Could you check a few things on this model? Use its own coordinates, in mm. Face numbers are marked on the shaded views. A direction names the side the tool comes from. Give positions to 0.01 mm unless a question says otherwise; leave off trailing zeros. Order: outer loops, then holes, each group sorted by start corner. A loop starts at its lowest first (then second) coordinate and runs counter-clockwise, first axis right, second up. Notation, with made-up numbers: M 26,-31 L 43,-31 A18 cw 43,-25 Z; hole C -24,-32 d2. An arc over 180 degrees is marked long. Use a Markdown table: item, result. Add a question column.
Item 1: If I drill on L1, parallel to X at y = -1078.5, z = -13.75; L2, parallel to Z at x = 811, y = -678; L3, parallel to X at y = -1253.5, z = -1.5, over which ranges is the centre line in solid material (lowest first)? Write a range as from..to.
Item 2: I'm going to push flat-ended pins straight in: pin 1 Ø1.6 at (y, z) = (-879, 1.5) entering from +X; pin 2 Ø4.5 at (y, z) = (-675.5, -10) entering from -X; pin 3 Ø1 at (x, y) = (842.5, -845.5) entering from -Z. Where does each tip first touch, or does it pass through?
Item 3: Suppose I cut it at C-C on y = -1213. Write out the boundary of the cut face in (x, z).
Item 4: Suppose I cut it at D-D on y = -548. Write out the boundary of the cut face in (x, z), plus the area to 3 significant figures.
Item 5: For the marked faces 1 and 2, which set-ups out of +Z, -Z, +X, -X, +Y, -Y let a thin tool reach every point of the face, with its end or its side?
Item 6: Suppose I cut it at A-A on z = -6.5. Write out the boundary of the cut face in (x, y), plus the area to 3 significant figures.
Item 7: Suppose I cut it at B-B on x = 830.5. Write out the boundary of the cut face in (y, z), plus the area to 3 significant figures.
Autodesk Inventor part; units mm, degrees
ref_plane "YZ Plane" through (0, 0, 0) normal (1, 0, 0) x (0, 1, 0)
ref_plane "XZ Plane" through (0, 0, 0) normal (0, 1, 0) x (-1, 0, 0)
ref_plane "XY Plane" through (0, 0, 0) normal (0, 0, 1) x (1, 0, 0)
sketch "Sketch1" plane through (0, 0, 0) normal (0, 0, 1) x (1, 0, 0)
  arc A0 (750, -2100) -> (770.3488, -241.0426) centre (-10250, -1050) ccw construction
  arc A1 (752.9864, -2100.2851) -> (771.4818, -215.8854) centre (-10246.9892, -1050.0296) ccw
  line L0 (-750, -2700) -> (-750, 0) construction
  line L1 (-800, 50) -> (-800, -2750) construction
  line L2 (-850, -2800) -> (-850, 100) construction
  line L3 (850, 100) -> (850, -2800)
  line L4 (800, -2750) -> (800, 50) construction
  line L5 (750, 0) -> (750, -2700) construction
  line L6 (770.3488, -241.0426) -> (767.3569, -241.2622) construction
  line L7 (768.4904, -216.1118) -> (771.4818, -215.8854) construction
  arc A2 (747.4657, -5.0326) -> (744.8748, -2.3426) centre (744.4792, -5.3164) ccw construction
  arc A3 (747.4657, -5.0326) -> (747.0136, -0.2851) centre (-10252.9895, -1050.2524) ccw construction
  arc A4 (767.3569, -241.2622) -> (747.4657, -5.0326) centre (-10252.9895, -1050.2524) ccw construction
  line L8 (750, 0) -> (747.0136, -0.2851) construction
  arc A5 (750.4522, -4.7486) -> (750, 0) centre (-10250, -1050) ccw construction
  arc A6 (750.4522, -4.7486) -> (745.2706, 0.6314) centre (744.4791, -5.3162) ccw
  line L9 (-750, 0) -> (750, 0) construction
  line L10 (-850, 100) -> (850, 100) construction
  line L11 (800, 50) -> (-800, 50) construction
  arc A7 (770.3488, -241.0426) -> (750.4522, -4.7486) centre (-10250, -1050) ccw
  line L12 (750, -2700) -> (-750, -2700) construction
  line L13 (750, -2100) -> (752.9864, -2100.2851) construction
  line L14 (-800, -2750) -> (800, -2750)
  line L15 (850, -2800) -> (-850, -2800) construction
  arc A8 (110, -2700) -> (114.1118, -2698.3696) centre (110, -2694) ccw construction
  line L16 (0, -2697) -> (110, -2697) construction
  line L17 (0, -2700) -> (0, -2697) construction
  arc A9 (750, 0) -> (745.2706, 0.6314) centre (0, -5600) ccw construction
  line L18 (750, 0) -> (749.6018, -2.9735) construction
  arc A10 (750, -3.0268) -> (0, 47) centre (-0.2, -5603) ccw construction
  line L19 (0, 47) -> (0, 0) construction
  line L20 (0, 50) -> (0, 47) construction
  line L21 (0, 100) -> (0, 50)
  arc A11 (745.2706, 0.6314) -> (0, 50) centre (0, -5600) ccw construction
  line L22 (-750, -2100) -> (750, -2100) construction
  arc A12 (110, -2697) -> (112.0559, -2696.1848) centre (110, -2694) ccw construction
  line L23 (676.3163, -2173.4556) -> (674.2605, -2171.2708) construction
  line L24 (690.4112, -2151.9536) -> (692.4671, -2154.1384) construction
  line L25 (752.0559, -2102.1848) -> (676.3163, -2173.4556) construction
  line L26 (114.1118, -2698.3696) -> (750, -2100) construction
  arc A13 (752.0559, -2102.1848) -> (752.9864, -2100.2851) centre (749.9998, -2099.9999) ccw construction
  line L27 (750, -2100) -> (752.0559, -2102.1848) construction
  arc A14 (749.1768, -2100.7746) -> (750.1074, -2098.8746) centre (747.1209, -2098.5898) ccw construction
  line L28 (112.0559, -2696.1848) -> (690.4112, -2151.9536) construction
  line L29 (850, -261.0426) -> (774.8074, -261.0426)
  arc A15 (800, 50) -> (0, 100) centre (0, -6325) ccw construction
  arc A16 (824.8074, -261.0426) -> (800, 50) centre (-10695.3477, -1023.3288) ccw construction
  line L30 (824.8074, -261.0426) -> (824.8074, 100) construction
  arc A17 (789.9065, -2131.1044) -> (824.8074, -261.0426) centre (-10201.0809, -990.6233) ccw construction
  line L31 (0, -2700) -> (0, -2750) construction
  line L32 (112.3791, -2700) -> (132.2053, -2750) construction
  line L33 (132.2053, -2750) -> (850, -2074.5565)
  arc A18 (770.2924, -241.0467) -> (766.5756, -191.1852) centre (768.4904, -216.1118) ccw construction
  line L34 (850, -400) -> (783.8749, -400) construction
  line L35 (850, -900) -> (801.9923, -900) construction
  line L36 (850, -1400) -> (797.4674, -1400) construction
  line L37 (850, -1900) -> (770.2723, -1900) construction
  line L38 (350, 100) -> (350, 39.1489)
  line L39 (-1472.612, -150) -> (-973.4947, -150)
  line L40 (-1472.612, -700) -> (-973.4947, -700)
  line L41 (-1472.612, -1250) -> (-973.4947, -1250)
  line L42 (-1472.612, -1800) -> (-973.4947, -1800)
  line L43 (800, -2750) -> (850, -2750) construction
  line L44 (752.9864, -2100.2851) -> (850, -2100.2851)
  point P0 (822.6583, -2100.2851)
  dimension "d16" = 1500
  dimension "d17" = 2700
  dimension "d18" = 2100
  dimension "d19" = 6
  dimension "d20" = 3
  dimension "d21" = 3
  dimension "d22" = 6
  dimension "d23" = 3
  dimension "d24" = 241.9
  dimension "d25" = 50
  dimension "d26" = 50
  dimension "d27" = 3
  dimension "d28" = 110
  dimension "d29" = 25
  dimension "d30" = 104
  dimension "d31" = 25
  dimension "d32" = 20
  dimension "d33" = 50
  dimension "d57" = 500
  dimension "d58" = 500
  dimension "d59" = 500
  dimension "d60" = 500
  dimension "d61" = 500
  dimension "d83" = 250
  dimension "d86" = 550
  dimension "d91" = 274.5565
extrude "Plate3" add sketch "Sketch1" along normal blind 2
sketch "Sketch3" plane through (848, -261.0426, 2) normal (1, 0, 0) x (0, 1, 0)
  line L0 (-1839.2425, 0) -> (0, 0)
  line L1 (0, 0) -> (0, 20)
  line L2 (0, 20) -> (-1839.2425, 20)
  line L3 (-1839.2425, 20) -> (-1839.2425, 0)
edge flange "Flange2" height 20 angle 90 thickness 2 bend radius 2.75 thickness toward (1, 0, 0) relief round relief width 2 relief depth 1 edges at (850, -1167.7996, 2) wall of the first edge with corners at (848, -2100.2851, 2) (848, -261.0426, 2) (848, -261.0426, -18) (848, -2100.2851, -18)
bend "Bend2"
corner "Corner2"
sketch "Sketch5" plane through (0, 0, 0) normal (0, 0, 1) x (1, 0, 0)
  line L0 (845.25, -2100.2851) -> (845.25, -261.0426)
  line L1 (774.8074, -261.0426) -> (845.25, -261.0426)
  arc A0 (752.9864, -2100.2851) -> (774.8074, -261.0426) centre (-10246.9892, -1050.0296) ccw
  line L2 (850, -261.0426) -> (850, -2100.2851)
  line L3 (850, -376.0426) -> (819, -376.0426)
  line L4 (850, -378.0426) -> (848, -378.0426) construction
  line L5 (848, -2100.2851) -> (848, -261.0426)
  line L6 (819, -376.0426) -> (819, -378.0426)
  line L7 (850, -876.0416) -> (801.641, -876.0416) construction
  line L8 (850, -878.0416) -> (801.6723, -878.0416) construction
  line L9 (820, -876.0416) -> (820, -878.0416) construction
  line L10 (850, -1376.0416) -> (798.2005, -1376.0416) construction
  line L11 (850, -1378.0416) -> (798.1413, -1378.0416) construction
  line L12 (820, -1376.0416) -> (820, -1378.0416) construction
  line L13 (850, -1876.0416) -> (772.0945, -1876.0416) construction
  line L14 (850, -1878.0416) -> (771.9443, -1878.0416) construction
  line L15 (820, -1876.0416) -> (820, -1878.0416) construction
  line L16 (850, -881.0416) -> (845.25, -881.0416) construction
  line L17 (845.25, -1381.0416) -> (850, -1381.0416) construction
  line L18 (845.25, -1881.0416) -> (850, -1881.0416) construction
  line L19 (845.25, -2100.2851) -> (752.9864, -2100.2851)
  line L20 (850, -376.0426) -> (850, -381.0426)
  line L21 (848, -376.0426) -> (848, -378.0426) construction
  line L22 (850, -381.0426) -> (848, -381.0426)
  line L23 (819, -376.0426) -> (782.437, -376.0426) construction
  line L24 (819, -378.0426) -> (782.559, -378.0426) construction
  line L25 (848, -378.0426) -> (848, -381.0426)
  line L26 (848, -378.0426) -> (819, -378.0426)
  line L27 (848, -381.0426) -> (845.25, -381.0426)
  point P0 (0, 0)
  point P1 (845.25, -380.4205)
  point P2 (848, -380.4205)
  point P3 (848, -1881.0416)
  point P4 (848, -1878.0416)
  point P5 (848, -1381.0416)
  point P6 (848, -1378.0416)
  point P7 (848, -881.0416)
  point P8 (848, -878.0416)
  point P9 (819, -377.0426)
  point P10 (848, -381.0426)
  point P11 (850, -410.4205)
  point P12 (848, -376.0426)
  point P13 (820, -877.0416)
  point P14 (820, -1377.0416)
  point P15 (820, -1877.0416)
  point P16 (848, -381.0426)
  point P17 (845.25, -378.0426)
  dimension "d69" = 1839.2425
  dimension "d70" = 2
  dimension "d76" = 67.563
  dimension "d80" = 48.359
  dimension "d81" = 30
  dimension "d94" = 5
  dimension "d95" = 30
  dimension "d96" = 5
  dimension "d97" = 30
  dimension "d98" = 5
  dimension "d102" = 77.9056
  dimension "d104" = 51.7995
  dimension "d106" = 2
  dimension "d107" = 5
  dimension "d108" = 116
  dimension "d109" = 500
  dimension "d110" = 500
  dimension "d111" = 500
  dimension "d112" = 31
extrude "Extrusion2" cut sketch "Sketch5" along normal through all both and the other way through all contours L0 L26 L5 L27 | L26 L6 L3 L0 | L0 L3 L5 L26 | L5 L3 L2 L22
chamfer "Chamfer2" [suppressed]
pattern_linear "Rectangular Pattern3" count 4 spacing 500 along (0, -1, 0) of "Extrusion2"
sketch "Sketch6" plane through (0, 0, 0) normal (0, 0, -1) x (-1, 0, 0)
  line L0 (-803.1643, -1276.0426) -> (-817.1643, -1276.0426) construction
  line L1 (-817.1643, -1276.0426) -> (-817.1643, -1076.0426) construction
  line L2 (-817.1643, -1076.0426) -> (-803.1643, -1076.0426) construction
  line L3 (-803.1643, -1076.0426) -> (-803.1643, -1276.0426) construction
  line L4 (-752.9864, -2100.2851) -> (-845.25, -2100.2851)
  line L5 (-803.1643, -1801.0426) -> (-803.1643, -1851.0426) construction
  line L6 (-803.1643, -1851.0426) -> (-815.1643, -1851.0426) construction
  line L7 (-815.1643, -1851.0426) -> (-815.1643, -1801.0426) construction
  line L8 (-815.1643, -1801.0426) -> (-803.1643, -1801.0426) construction
  line L9 (-845.25, -1876.0426) -> (-819, -1876.0426)
  line L10 (-803.1643, -1301.0426) -> (-803.1643, -1351.0426) construction
  line L11 (-803.1643, -1351.0426) -> (-815.1643, -1351.0426) construction
  line L12 (-815.1643, -1351.0426) -> (-815.1643, -1301.0426) construction
  line L13 (-815.1643, -1301.0426) -> (-803.1643, -1301.0426) construction
  line L14 (-803.1643, -801.0426) -> (-803.1643, -851.0426) construction
  line L15 (-803.1643, -851.0426) -> (-815.1643, -851.0426) construction
  line L16 (-815.1643, -851.0426) -> (-815.1643, -801.0426) construction
  line L17 (-815.1643, -801.0426) -> (-803.1643, -801.0426) construction
  line L18 (-803.1643, -301.0426) -> (-803.1643, -351.0426) construction
  line L19 (-803.1643, -351.0426) -> (-815.1643, -351.0426) construction
  line L20 (-815.1643, -351.0426) -> (-815.1643, -301.0426) construction
  line L21 (-815.1643, -301.0426) -> (-803.1643, -301.0426) construction
  line L22 (-845.25, -1376.0426) -> (-819, -1376.0426)
  line L23 (-845.25, -876.0426) -> (-819, -876.0426)
  line L24 (-845.25, -376.0426) -> (-819, -376.0426)
  point P0 (0, 0)
  point P1 (-753.1643, -2098.4205)
  point P2 (-824.6397, -2098.4205)
  dimension "d120" = 200
  dimension "d121" = 14
  dimension "d124" = 50
  dimension "d125" = 12
  dimension "d126" = 50
  dimension "d127" = 25
  dimension "d128" = 50
  dimension "d129" = 12
  dimension "d130" = 50
  dimension "d131" = 12
  dimension "d132" = 50
  dimension "d133" = 12
  dimension "d134" = 50
  dimension "d135" = 25
  dimension "d136" = 25
  dimension "d137" = 25
  dimension "d138" = 50
  dimension "d139" = 50
  dimension "d140" = 50
  dimension "d143" = 100
mark "Mark1"
sketch "Sketch7" plane through (0, 0, 0) normal (0, 0, 1) x (1, 0, 0)
  line L0 (845.25, -1878.0426) -> (819, -1878.0426) construction
  line L1 (819, -1878.0426) -> (819, -1876.0426) construction
  line L2 (819, -1876.0426) -> (845.25, -1876.0426) construction
  line L3 (845.25, -1876.0426) -> (845.25, -1381.0426) construction
  line L4 (845.25, -1381.0426) -> (845.25, -1378.0426) construction
  line L5 (845.25, -1378.0426) -> (819, -1378.0426) construction
  line L6 (819, -1378.0426) -> (819, -1376.0426) construction
  line L7 (819, -1376.0426) -> (845.25, -1376.0426) construction
  line L8 (845.25, -1376.0426) -> (845.25, -881.0426) construction
  line L9 (845.25, -881.0426) -> (845.25, -878.0426) construction
  line L10 (845.25, -878.0426) -> (819, -878.0426) construction
  line L11 (819, -878.0426) -> (819, -876.0426) construction
  line L12 (819, -876.0426) -> (845.25, -876.0426) construction
  line L13 (845.25, -876.0426) -> (845.25, -381.0426) construction
  line L14 (845.25, -381.0426) -> (845.25, -378.0426)
  line L15 (845.25, -378.0426) -> (819, -378.0426)
  line L16 (819, -378.0426) -> (819, -376.0426)
  line L17 (819, -376.0426) -> (845.25, -376.0426)
  line L18 (845.25, -376.0426) -> (845.25, -261.0426)
  line L19 (774.8074, -261.0426) -> (845.25, -261.0426)
  arc A0 (752.9864, -2100.2851) -> (774.8074, -261.0426) centre (-10246.9892, -1050.0296) ccw construction
  line L20 (845.25, -2100.2851) -> (752.9864, -2100.2851) construction
  line L21 (845.25, -2100.2851) -> (845.25, -1881.0426) construction
  line L22 (845.25, -1881.0426) -> (845.25, -1878.0426) construction
  line L23 (716.6808, -2132.1957) -> (990.5996, -2132.1957)
  line L24 (990.5996, -2132.1957) -> (990.5996, -1376.0426)
  line L25 (990.5996, -1376.0426) -> (716.6808, -1376.0426)
  line L26 (716.6808, -1376.0426) -> (716.6808, -2132.1957)
  point P0 (0, 0)
extrude "Extrusion3" cut sketch "Sketch7" along normal through all both and the other way through all
equation "\"d16\" = d34"
equation "\"d17\" = d35"
equation "\"d18\" = d36"
equation "\"d19\" = d37"
equation "\"d20\" = d38"
equation "\"d21\" = d39"
equation "\"d22\" = d39 + d43"
equation "\"d23\" = d39"
equation "\"d27\" = d39"
equation "\"d28\" = 0.5 * d44"
equation "\"d29\" = d41"
equation "\"d30\" = d42"
equation "\"d31\" = d41"
equation "\"d33\" = d25"
equation "\"Стрингер_3\" = 67.36301"
equation "\"d37\" = d39 + d43"
equation "\"d38\" = d39"
equation "\"d43\" = d39"
equation "\"Стрингер_4\" = 48.15903"
equation "\"Стрингер_5\" = 51.59945"
equation "\"Стрингер_6\" = 77.70555"
properties part number "MSC 315 rib hip" material "Stainless Steel"
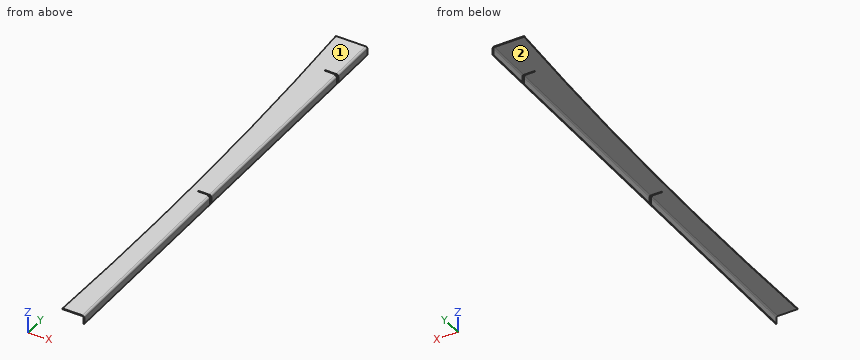
Findings below:
| question | item | result |
|---|---|---|
| 1 | L1 | x = 848..850 |
| 1 | L2 | z = 0..2 |
| 1 | L3 | x = 847.7..849.83 |
| 2 | pin 1 | stops at x = 845.25 |
| 2 | pin 2 | stops at x = 848 |
| 2 | pin 3 | stops at z = 0 |
| 3 | outline | M 801.81,0 L 845.25,0 A2.75 cw 848,-2.75 L 848,-18 L 850,-18 L 850,-2.75 A4.75 ccw 845.25,2 L 801.81,2 Z |
| 4 | outline | M 791.6,0 L 845.25,0 A2.75 cw 848,-2.75 L 848,-18 L 850,-18 L 850,-2.75 A4.75 ccw 845.25,2 L 791.6,2 Z |
| 4 | area | 150 mm^2 |
| 5 | face 1 | +Z, +X, -X, +Y, -Y |
| 5 | face 2 | -Z, -X, +Y, -Y |
| 6 | outline | M 848,-1376.04 L 850,-1376.04 L 850,-881.04 L 848,-881.04 Z; M 848,-876.04 L 850,-876.04 L 850,-381.04 L 848,-381.04 Z; M 848,-376.04 L 850,-376.04 L 850,-261.04 L 848,-261.04 Z |
| 6 | area | 2,210 mm^2 |
| 7 | outline | M -1376.04,0 L -878.04,0 L -878.04,2 L -1376.04,2 Z; M -876.04,0 L -378.04,0 L -378.04,2 L -876.04,2 Z; M -376.04,0 L -261.04,0 L -261.04,2 L -376.04,2 Z |
| 7 | area | 2,220 mm^2 |
